Autodesk Fusion 360 part; units mm, degrees
sketch "3x8-Edge_Cuts" plane through (0, 0, 0) normal (0, 0, 1) x (1, 0, 0)
  line L0 (17, -29.5) -> (17, -100.6)
  line L1 (17, -100.6) -> (193, -100.6)
  line L2 (193, -29.5) -> (17, -29.5)
  line L3 (193, -100.6) -> (193, -29.5)
sketch "3x8-User_Comments" plane through (0, 0, 0) normal (0, 0, 1) x (1, 0, 0)
  circle A0 centre (105.98, -53.92) radius 3
  circle A1 centre (39.54, -54.16) radius 3
  circle A2 centre (170.85, -54.72) radius 3
sketch "3x8-User_Drawings" plane through (0, 0, 0) normal (0, 0, 1) x (1, 0, 0)
  circle A0 centre (138.077, -65.15) radius 9
  circle A1 centre (28.0768, -41.45) radius 9
  circle A2 centre (138.077, -88.85) radius 9
  circle A3 centre (72.0768, -88.85) radius 9
  circle A4 centre (116.077, -88.85) radius 9
  circle A5 centre (50.0768, -41.45) radius 9
  circle A6 centre (94.0768, -41.45) radius 9
  circle A7 centre (160.077, -88.85) radius 9
  circle A8 centre (72.0768, -41.45) radius 9
  circle A9 centre (138.077, -41.45) radius 9
  circle A10 centre (50.0768, -65.15) radius 9
  circle A11 centre (28.0768, -88.85) radius 9
  circle A12 centre (116.077, -41.45) radius 9
  circle A13 centre (94.0768, -88.85) radius 9
  circle A14 centre (28.0768, -65.15) radius 9
  circle A15 centre (116.077, -65.15) radius 9
  circle A16 centre (160.077, -41.45) radius 9
  circle A17 centre (160.077, -65.15) radius 9
  circle A18 centre (50.0768, -88.85) radius 9
  circle A19 centre (94.0768, -65.15) radius 9
  circle A20 centre (182.077, -65.15) radius 9
  circle A21 centre (182.077, -41.45) radius 9
  circle A22 centre (182.077, -88.85) radius 9
  circle A23 centre (72.0768, -65.15) radius 9
extrude "Extrude1" add sketch "3x8-Edge_Cuts" along normal blind 2
extrude "Extrude2" cut sketch "3x8-User_Drawings" sketch "3x8-User_Comments" along normal blind 2 of sketch 2
Work out the finished part from the listing and answer in its coordinate system (mm). Round coordinates to 2 decimals unless told otherwise and drop trailing zeros. Write each loop counter-clockwise with the first axis right and the second up, starting at its lowest first coordinate (ties: lowest second). Pieces come first, ordered by that corner, then holes. Notation, with made-up numbers: M 11.25,-38.5 L 46.25,-38.5 A29 cw 46.25,-0.5 Z; hole C 88.25,-14.5 d5. An arc over 180 degrees is marked long. Use a Markdown table: item, result.
1) Consider line 1 (Y direction, x = 52, z = 0.55); line 2 (Y direction, x = 66, z = 0.5); line 3 (Y direction, x = 106, z = 1.8). Determine where each line is inside the solid, lowest interval first. Write a range as [from, to].
Taken from the geometry:
| item | result |
|---|---|
| line 1 | y = [-100.6, -97.64], [-80.06, -73.94], [-56.36, -50.24], [-32.66, -29.5] |
| line 2 | y = [-100.6, -95.49], [-82.21, -71.79], [-58.51, -48.09], [-34.81, -29.5] |
| line 3 | y = [-100.6, -56.92], [-50.92, -29.5] |
2) The part is cut by section B-B on z = 1.45. State how many separate pieces and enclosed holes the cut face has, plus the area to 3 significant figures.
Taken from the geometry:
| item | result |
|---|---|
| separate pieces | 1 |
| enclosed holes | 27 |
| area | 6,320 mm2 |
3) Determine the mould class of faces 1 (the face through (104, -65, 0)), 2 (the face through (172.234, -52.058, 0.986)) for opening direction X: pulls with the +X half, pulls with the -X half, needs draft (parallel to the pull), parting line crosses it, or undercut.
Taken from the geometry:
| item | result |
|---|---|
| face 1 | needs draft |
| face 2 | undercut |
4) The part is cut by section C-C on x = 123.5. Give the vertices of the cut face in (y, z).
Taken from the geometry:
| item | result |
|---|---|
| outline | M -100.6,0 L -93.94,0 L -93.94,2 L -100.6,2 Z; M -83.76,0 L -70.24,0 L -70.24,2 L -83.76,2 Z; M -60.06,0 L -46.54,0 L -46.54,2 L -60.06,2 Z; M -36.36,0 L -29.5,0 L -29.5,2 L -36.36,2 Z |
5) The part is cut by section A-A on x = 39.54. Give the vertices of the cut face in (y, z).
Taken from the geometry:
| item | result |
|---|---|
| outline | M -100.6,0 L -57.16,0 L -57.16,2 L -100.6,2 Z; M -51.16,0 L -29.5,0 L -29.5,2 L -51.16,2 Z |
